Work out the finished part from the listing and answer in its coordinate system (mm). Face numbers are marked on the shaded views. A direction names the side the tool comes from. Give positions to 0.01 mm unless a question says otherwise; leave off trailing zeros. Write each loop counter-clockwise with the first axis right and the second up, starting at its lowest first coordinate (ties: lowest second). Pieces come first, ordered by that corner, then holes.
1) Find section A-A (y = 52.5). Determine the outline of the cut face in (x, z), plus the area to 3 significant figures.
2) Find section B-B (x = 62.5). Determine the outline of the cut face in (y, z).
3) Determine the mould class of the marked faces 1, 2 and 3 for opening direction Y: pulls with the +Y half, pulls with the -Y half, needs draft (parallel to the pull), parting line crosses it, or undercut.
4) Find section C-C (z = 8). Determine the outline of the cut face in (x, y).
5) Given pin 1 Ø6.5 at (x, y) = (63.5, 29.5) entering from +Z; pin 2 Ø24 at (x, y) = (27.5, 22.5) entering from +Z; pin 3 Ø3 at (x, y) = (62.5, 52.5) entering from +Z; pin 4 Ø1.5 at (y, z) = (36, 7.5) entering from +X, each flat-ended and moving along its own axis, determine where each tip first touches the part or whether it passes through.
6) Find section D-D (z = 3). Determine the outline of the cut face in (x, y), plus the area to 3 significant figures.
7) Straight lines are drawn through the part: probe 1 along Y at (x, z) = (62.5, 3.25); probe 2 along Y at (x, z) = (62.5, 6.75); probe 3 along X at (y, z) = (37.5, 3). For each, find the intervals that lie inside material, in ascending order.
8) A tool of negligible diameter and unlimited length cuts with its end or side. For the marked faces 4 and 5, from which of +Z, -Z, +X, -X, +Y, -Y can it reach the whole face along a straight path? Write none if from no direction.
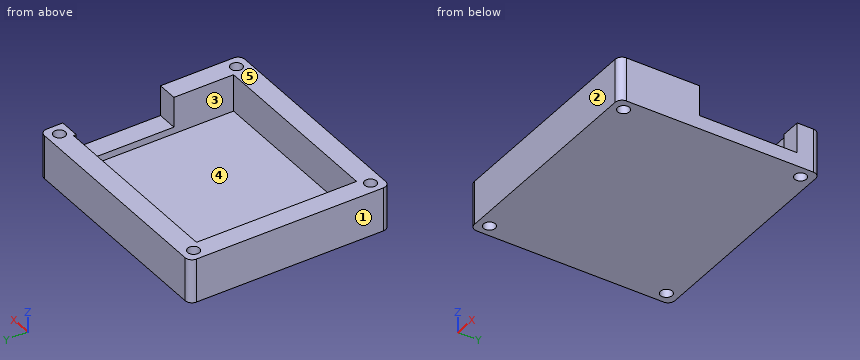
Autodesk Fusion 360 part; units mm, degrees
sketch "Sketch1" plane through (0, 0, 0) normal (0, 0, 1) x (1, 0, 0)
  line L0 (4.874, 50) -> (60, 50)
  line L1 (60, 50) -> (60, 2.5)
  line L2 (60, 2.5) -> (4.874, 2.5)
  line L3 (4.874, 2.5) -> (4.874, 50)
  line L4 (-1.126, 56) -> (66, 56)
  line L5 (66, 56) -> (66, -3.5)
  line L6 (66, -3.5) -> (-1.126, -3.5)
  line L7 (-1.126, -3.5) -> (-1.126, 56)
  circle A0 centre (2.374, 52.5) radius 1.75
  circle A1 centre (2.374, 0) radius 1.75
  circle A2 centre (62.5, 52.5) radius 1.75
  circle A3 centre (62.5, 0) radius 1.75
  dimension "d1" = 55.126
  dimension "d2" = 47.5
  dimension "d3" = 6
  dimension "d4" = 6
  dimension "d5" = 6
  dimension "d6" = 6
  dimension "d7" = 3.5
  dimension "d8" = 3.5
  dimension "d9" = 3.5
  dimension "d10" = 3.5
  dimension "d11" = 3.5
  dimension "d12" = 3.5
  dimension "d13" = 3.5
  dimension "d14" = 3.5
  dimension "d15" = 3.5
  dimension "d16" = 3.5
  dimension "d17" = 3.5
  dimension "d18" = 3.5
extrude "Extrude1" add sketch "Sketch1" along normal blind 13
extrude "Extrude2" add sketch "Sketch1" along normal blind 2 contours L0 L1 L2 L3
sketch "Sketch2" plane through (0, 0, 13) normal (0, 0, 1) x (-1, 0, 0)
  line L0 (-60, -2.5) -> (-4.874, -2.5)
  line L1 (-4.874, -2.5) -> (-4.874, -50)
  line L2 (-4.874, -50) -> (-60, -50)
  line L3 (-60, -50) -> (-60, -2.5)
  circle A0 centre (-62.5, -52.5) radius 1.75
  circle A1 centre (-2.374, -52.5) radius 1.75
  circle A2 centre (-2.374, 0) radius 1.75
  circle A3 centre (-62.5, 0) radius 1.75
  line L4 (1.126, 3.5) -> (-66, 3.5)
  line L5 (-66, 3.5) -> (-66, -56)
  line L6 (-66, -56) -> (1.126, -56)
  line L7 (1.126, -56) -> (1.126, 3.5)
  line L8 (-60, -49.1938) -> (-66, -49.1938)
  line L9 (-66, -49.1938) -> (-66, -20.1938)
  line L10 (-66, -20.1938) -> (-60, -20.1938)
  line L11 (-60, -20.1938) -> (-60, -49.1938)
  dimension "d23" = 29
extrude "Extrude3" cut sketch "Sketch2" against normal blind 9 contours L3 L5 L8 L9 L10 L11
fillet "Fillet1" radius 2 4 edges at (-1.126, 56, 6.5) (-1.126, -3.5, 6.5) (66, -3.5, 6.5) (66, 56, 6.5)
Results:
1. outline: (-1.13, 0) - (0.62, 0) - (0.62, 13) - (-1.13, 13) - close; (4.12, 0) - (60.75, 0) - (60.75, 13) - (4.12, 13) - close; (64.25, 0) - (66, 0) - (66, 13) - (64.25, 13) - close
1. area: 782 mm2
2. outline: (-3.5, 0) - (-1.75, 0) - (-1.75, 13) - (-3.5, 13) - close; (1.75, 0) - (50.75, 0) - (50.75, 13) - (49.19, 13) - (49.19, 4) - (20.19, 4) - (20.19, 13) - (1.75, 13) - close; (54.25, 0) - (56, 0) - (56, 13) - (54.25, 13) - close
3. face 1: needs draft
3. face 2: pulls with the -Y half
3. face 3: undercut
4. outline: (-1.13, -1.5) arc R2 ccw to (0.87, -3.5) - (64, -3.5) arc R2 ccw to (66, -1.5) - (66, 20.19) - (60, 20.19) - (60, 2.5) - (4.87, 2.5) - (4.87, 50) - (60, 50) - (60, 49.19) - (66, 49.19) - (66, 54) arc R2 ccw to (64, 56) - (0.87, 56) arc R2 ccw to (-1.13, 54) - close; hole circle Ø3.5 at (2.37, 0); hole circle Ø3.5 at (2.37, 52.5); hole circle Ø3.5 at (62.5, 0); hole circle Ø3.5 at (62.5, 52.5)
5. pin 1: stops at z = 4
5. pin 2: stops at z = 2
5. pin 3: passes through
5. pin 4: stops at x = 4.87
6. outline: (-1.13, -1.5) arc R2 ccw to (0.87, -3.5) - (64, -3.5) arc R2 ccw to (66, -1.5) - (66, 54) arc R2 ccw to (64, 56) - (0.87, 56) arc R2 ccw to (-1.13, 54) - close; hole circle Ø3.5 at (2.37, 0); hole circle Ø3.5 at (2.37, 52.5); hole (4.87, 2.5) - (60, 2.5) - (60, 50) - (4.87, 50) - close; hole circle Ø3.5 at (62.5, 0); hole circle Ø3.5 at (62.5, 52.5)
6. area: 1,330 mm2
7. probe 1: y = -3.5 to -1.75, 1.75 to 50.75, 54.25 to 56
7. probe 2: y = -3.5 to -1.75, 1.75 to 20.19, 49.19 to 50.75, 54.25 to 56
7. probe 3: x = -1.13 to 4.87, 60 to 66
8. face 4: +Z
8. face 5: +Z, +X, -X, +Y, -Y
